Can you work these out from the model? Positions are in its coordinate system, mm. A direction names the side the tool comes from. Give positions to 0.01 mm unless a question says otherwise; leave off trailing zeros. Loops run counter-clockwise (first coordinate to the right, second up) from the corner with the lowest first, then second, coordinate; pieces in that order, holes last. Notation, with made-up numbers: (-4, 17) -> (15, 17) arc R8 cw to (15, 28) -> close; hole circle Ø5 at (-31.5, -15). An arc over 180 degrees is marked (long way). Use CSV: the item, a comma, the result in double quotes.
from build123d import *

# Parameters (mm, degrees)
F0_W     = 190
F0_H     = 60
F1_DEPTH = 5
F2_W     = 25
F2_H     = 20
F2_H_2   = 10
F2_W_2   = 24.9426496029
F3_DEPTH = 2
F4_W     = 25
F4_H     = 20
F4_H_2   = 10
F5_DEPTH = 2


with BuildPart() as f1:
    # F0 (on Top) → F1 (new body)
    with BuildSketch(Plane.XY):
        Rectangle(F0_W, F0_H)
        with BuildLine():
            Line((27, -16.5), (-27, -16.5))
            ThreePointArc((-27, -16.5), (-27.8535533906, -16.8535533906), (-27.5, -16))
            Line((-27.5, -16), (-27.5, -10))
            Line((-27.5, -10), (-42.4774698913, -10))
            Line((-42.4774698913, -10), (-42.4774698913, 10))
            Line((-42.4774698913, 10), (-27.5, 10))
            Line((-27.5, 10), (-27.5, 16))
            ThreePointArc((-27.5, 16), (-27.8535533906, 16.8535533906), (-27, 16.5))
            Line((-27, 16.5), (27, 16.5))
            ThreePointArc((27, 16.5), (27.5, 17), (28, 16.5))
            ThreePointArc((28, 16.5), (27.8535533906, 16.1464466094), (27.5, 16))
            Line((27.5, 16), (27.5, -16))
            ThreePointArc((27.5, -16), (27.8535533906, -16.1464466094), (28, -16.5))
            ThreePointArc((28, -16.5), (27.5, -17), (27, -16.5))
        make_face(mode=Mode.SUBTRACT)
        with BuildLine():
            ThreePointArc((-27.5, -16), (-27.1464466094, -16.1464466094), (-27, -16.5))
            Line((-27, -16.5), (27, -16.5))
            ThreePointArc((27, -16.5), (27.1464466094, -16.1464466094), (27.5, -16))
            Line((27.5, -16), (27.5, 16))
            ThreePointArc((27.5, 16), (27.1464466094, 16.1464466094), (27, 16.5))
            Line((27, 16.5), (-27, 16.5))
            ThreePointArc((-27, 16.5), (-27.1464466094, 16.1464466094), (-27.5, 16))
            Line((-27.5, 16), (-27.5, 10))
            Line((-27.5, 10), (-27.4774698913, 10))
            Line((-27.4774698913, 10), (-27.4774698913, -10))
            Line((-27.4774698913, -10), (-27.5, -10))
            Line((-27.5, -10), (-27.5, -16))
        make_face()
    extrude(amount=F1_DEPTH)

    # F2 (on face) → F3 (join)
    with BuildSketch(Plane.XY.offset(5)):
        Polygon((-95, -30), (-95, -20), (-95.0573503971, -20), (-95.0573503971, -50), (-70.0573503971, -50), (-70.0573503971, -30), align=None)
        with BuildLine():
            Line((-76.0573503971, -45), (-89.0573503971, -45))
            ThreePointArc((-89.0573503971, -45), (-90.7644571783, -45.7071067812), (-90.0573503971, -44))
            Line((-90.0573503971, -44), (-90.0573503971, -36))
            ThreePointArc((-90.0573503971, -36), (-90.7644571783, -34.2928932188), (-89.0573503971, -35))
            Line((-89.0573503971, -35), (-76.0573503971, -35))
            ThreePointArc((-76.0573503971, -35), (-75.0573503971, -34), (-74.0573503971, -35))
            ThreePointArc((-74.0573503971, -35), (-74.3502436159, -35.7071067812), (-75.0573503971, -36))
            Line((-75.0573503971, -36), (-75.0573503971, -44))
            ThreePointArc((-75.0573503971, -44), (-74.3502436159, -44.2928932188), (-74.0573503971, -45))
            ThreePointArc((-74.0573503971, -45), (-75.0573503971, -46), (-76.0573503971, -45))
        make_face(mode=Mode.SUBTRACT)
        with Locations((-82.5, 40)):
            Rectangle(F2_W, F2_H)
        with BuildLine():
            ThreePointArc((-90, 44), (-90.7071067812, 45.7071067812), (-89, 45))
            Line((-89, 45), (-76, 45))
            ThreePointArc((-76, 45), (-75, 46), (-74, 45))
            ThreePointArc((-74, 45), (-74.2928932188, 44.2928932188), (-75, 44))
            Line((-75, 44), (-75, 36))
            ThreePointArc((-75, 36), (-74.2928932188, 35.7071067812), (-74, 35))
            ThreePointArc((-74, 35), (-75, 34), (-76, 35))
            Line((-76, 35), (-89, 35))
            ThreePointArc((-89, 35), (-90.7071067812, 34.2928932188), (-90, 36))
            Line((-90, 36), (-90, 44))
        make_face(mode=Mode.SUBTRACT)
        with Locations((82.5, 40)):
            Rectangle(F2_W, F2_H)
        with BuildLine():
            ThreePointArc((75, 44), (74.2928932188, 45.7071067812), (76, 45))
            Line((76, 45), (89, 45))
            ThreePointArc((89, 45), (90, 46), (91, 45))
            ThreePointArc((91, 45), (90.7071067812, 44.2928932188), (90, 44))
            Line((90, 44), (90, 36))
            ThreePointArc((90, 36), (90.7071067812, 35.7071067812), (91, 35))
            ThreePointArc((91, 35), (90, 34), (89, 35))
            Line((89, 35), (76, 35))
            ThreePointArc((76, 35), (74.2928932188, 34.2928932188), (75, 36))
            Line((75, 36), (75, 44))
        make_face(mode=Mode.SUBTRACT)
        with Locations((82.5, -40)):
            Rectangle(F2_W, F2_H)
        with BuildLine():
            Line((89, -45), (76, -45))
            ThreePointArc((76, -45), (74.2928932188, -45.7071067812), (75, -44))
            Line((75, -44), (75, -36))
            ThreePointArc((75, -36), (74.2928932188, -34.2928932188), (76, -35))
            Line((76, -35), (89, -35))
            ThreePointArc((89, -35), (90, -34), (91, -35))
            ThreePointArc((91, -35), (90.7071067812, -35.7071067812), (90, -36))
            Line((90, -36), (90, -44))
            ThreePointArc((90, -44), (90.7071067812, -44.2928932188), (91, -45))
            ThreePointArc((91, -45), (90, -46), (89, -45))
        make_face(mode=Mode.SUBTRACT)
        with Locations((-82.5, 25)):
            Rectangle(F2_W, F2_H_2)
        with Locations((82.5, 25)):
            Rectangle(F2_W, F2_H_2)
        with Locations((82.5, -25)):
            Rectangle(F2_W, F2_H_2)
        with Locations((-82.5286751986, -25)):
            Rectangle(F2_W_2, F2_H_2)
        with BuildLine():
            Line((-76, 45), (-89, 45))
            ThreePointArc((-89, 45), (-89.2928932188, 44.2928932188), (-90, 44))
            Line((-90, 44), (-90, 36))
            ThreePointArc((-90, 36), (-89.2928932188, 35.7071067812), (-89, 35))
            Line((-89, 35), (-76, 35))
            ThreePointArc((-76, 35), (-75.7071067812, 35.7071067812), (-75, 36))
            Line((-75, 36), (-75, 44))
            ThreePointArc((-75, 44), (-75.7071067812, 44.2928932188), (-76, 45))
        make_face()
        with BuildLine():
            Line((89, 45), (76, 45))
            ThreePointArc((76, 45), (75.7071067812, 44.2928932188), (75, 44))
            Line((75, 44), (75, 36))
            ThreePointArc((75, 36), (75.7071067812, 35.7071067812), (76, 35))
            Line((76, 35), (89, 35))
            ThreePointArc((89, 35), (89.2928932188, 35.7071067812), (90, 36))
            Line((90, 36), (90, 44))
            ThreePointArc((90, 44), (89.2928932188, 44.2928932188), (89, 45))
        make_face()
        with BuildLine():
            ThreePointArc((75, -44), (75.7071067812, -44.2928932188), (76, -45))
            Line((76, -45), (89, -45))
            ThreePointArc((89, -45), (89.2928932188, -44.2928932188), (90, -44))
            Line((90, -44), (90, -36))
            ThreePointArc((90, -36), (89.2928932188, -35.7071067812), (89, -35))
            Line((89, -35), (76, -35))
            ThreePointArc((76, -35), (75.7071067812, -35.7071067812), (75, -36))
            Line((75, -36), (75, -44))
        make_face()
        with BuildLine():
            ThreePointArc((-90.0573503971, -44), (-89.3502436159, -44.2928932188), (-89.0573503971, -45))
            Line((-89.0573503971, -45), (-76.0573503971, -45))
            ThreePointArc((-76.0573503971, -45), (-75.7644571783, -44.2928932188), (-75.0573503971, -44))
            Line((-75.0573503971, -44), (-75.0573503971, -36))
            ThreePointArc((-75.0573503971, -36), (-75.7644571783, -35.7071067812), (-76.0573503971, -35))
            Line((-76.0573503971, -35), (-89.0573503971, -35))
            ThreePointArc((-89.0573503971, -35), (-89.3502436159, -35.7071067812), (-90.0573503971, -36))
            Line((-90.0573503971, -36), (-90.0573503971, -44))
        make_face()
    extrude(amount=F3_DEPTH)

    # F4 (on face) → F5 (join)
    with BuildSketch(Plane(origin=(0, 0, 0), x_dir=(1, 0, 0), z_dir=(0, 0, -1))):
        with Locations((-82.5, 40)):
            Rectangle(F4_W, F4_H)
        with BuildLine():
            ThreePointArc((-90, 44), (-90.7071067812, 45.7071067812), (-89, 45))
            Line((-89, 45), (-76, 45))
            ThreePointArc((-76, 45), (-75, 46), (-74, 45))
            ThreePointArc((-74, 45), (-74.2928932188, 44.2928932188), (-75, 44))
            Line((-75, 44), (-75, 36))
            ThreePointArc((-75, 36), (-74.2928932188, 35.7071067812), (-74, 35))
            ThreePointArc((-74, 35), (-75, 34), (-76, 35))
            Line((-76, 35), (-89, 35))
            ThreePointArc((-89, 35), (-90.7071067812, 34.2928932188), (-90, 36))
            Line((-90, 36), (-90, 44))
        make_face(mode=Mode.SUBTRACT)
        with Locations((82.5, 40)):
            Rectangle(F4_W, F4_H)
        with BuildLine():
            ThreePointArc((75, 44), (74.2928932188, 45.7071067812), (76, 45))
            Line((76, 45), (89, 45))
            ThreePointArc((89, 45), (90, 46), (91, 45))
            ThreePointArc((91, 45), (90.7071067812, 44.2928932188), (90, 44))
            Line((90, 44), (90, 36))
            ThreePointArc((90, 36), (90.7071067812, 35.7071067812), (91, 35))
            ThreePointArc((91, 35), (90, 34), (89, 35))
            Line((89, 35), (76, 35))
            ThreePointArc((76, 35), (74.2928932188, 34.2928932188), (75, 36))
            Line((75, 36), (75, 44))
        make_face(mode=Mode.SUBTRACT)
        with Locations((82.5, -40)):
            Rectangle(F4_W, F4_H)
        with BuildLine():
            Line((89, -45), (76, -45))
            ThreePointArc((76, -45), (74.2928932188, -45.7071067812), (75, -44))
            Line((75, -44), (75, -36.0721963992))
            ThreePointArc((75, -36.0721963992), (74.2928932188, -34.365089618), (76, -35.0721963992))
            Line((76, -35.0721963992), (89, -35.0721963992))
            ThreePointArc((89, -35.0721963992), (90, -34.0721963992), (91, -35.0721963992))
            ThreePointArc((91, -35.0721963992), (90.7071067812, -35.7793031804), (90, -36.0721963992))
            Line((90, -36.0721963992), (90, -44))
            ThreePointArc((90, -44), (90.7071067812, -44.2928932188), (91, -45))
            ThreePointArc((91, -45), (90, -46), (89, -45))
        make_face(mode=Mode.SUBTRACT)
        with Locations((-82.5, -40)):
            Rectangle(F4_W, F4_H)
        with BuildLine():
            Line((-76, -45), (-89, -45))
            ThreePointArc((-89, -45), (-90.7071067812, -45.7071067812), (-90, -44))
            Line((-90, -44), (-90, -36))
            ThreePointArc((-90, -36), (-90.7071067812, -34.2928932188), (-89, -35))
            Line((-89, -35), (-76, -35))
            ThreePointArc((-76, -35), (-75, -34), (-74, -35))
            ThreePointArc((-74, -35), (-74.2928932188, -35.7071067812), (-75, -36))
            Line((-75, -36), (-75, -44))
            ThreePointArc((-75, -44), (-74.2928932188, -44.2928932188), (-74, -45))
            ThreePointArc((-74, -45), (-75, -46), (-76, -45))
        make_face(mode=Mode.SUBTRACT)
        with Locations((-82.5, 25)):
            Rectangle(F4_W, F4_H_2)
        with Locations((82.5, 25)):
            Rectangle(F4_W, F4_H_2)
        with Locations((82.5, -25)):
            Rectangle(F4_W, F4_H_2)
        with Locations((-82.5, -25)):
            Rectangle(F4_W, F4_H_2)
        with BuildLine():
            Line((-76, 45), (-89, 45))
            ThreePointArc((-89, 45), (-89.2928932188, 44.2928932188), (-90, 44))
            Line((-90, 44), (-90, 36))
            ThreePointArc((-90, 36), (-89.2928932188, 35.7071067812), (-89, 35))
            Line((-89, 35), (-76, 35))
            ThreePointArc((-76, 35), (-75.7071067812, 35.7071067812), (-75, 36))
            Line((-75, 36), (-75, 44))
            ThreePointArc((-75, 44), (-75.7071067812, 44.2928932188), (-76, 45))
        make_face()
        with BuildLine():
            Line((89, 45), (76, 45))
            ThreePointArc((76, 45), (75.7071067812, 44.2928932188), (75, 44))
            Line((75, 44), (75, 36))
            ThreePointArc((75, 36), (75.7071067812, 35.7071067812), (76, 35))
            Line((76, 35), (89, 35))
            ThreePointArc((89, 35), (89.2928932188, 35.7071067812), (90, 36))
            Line((90, 36), (90, 44))
            ThreePointArc((90, 44), (89.2928932188, 44.2928932188), (89, 45))
        make_face()
        with BuildLine():
            ThreePointArc((-90, -44), (-89.2928932188, -44.2928932188), (-89, -45))
            Line((-89, -45), (-76, -45))
            ThreePointArc((-76, -45), (-75.7071067812, -44.2928932188), (-75, -44))
            Line((-75, -44), (-75, -36))
            ThreePointArc((-75, -36), (-75.7071067812, -35.7071067812), (-76, -35))
            Line((-76, -35), (-89, -35))
            ThreePointArc((-89, -35), (-89.2928932188, -35.7071067812), (-90, -36))
            Line((-90, -36), (-90, -44))
        make_face()
        with BuildLine():
            ThreePointArc((75, -44), (75.7071067812, -44.2928932188), (76, -45))
            Line((76, -45), (89, -45))
            ThreePointArc((89, -45), (89.2928932188, -44.2928932188), (90, -44))
            Line((90, -44), (90, -36.0721963992))
            ThreePointArc((90, -36.0721963992), (89.2928932188, -35.7793031804), (89, -35.0721963992))
            Line((89, -35.0721963992), (76, -35.0721963992))
            ThreePointArc((76, -35.0721963992), (75.7071067812, -35.7793031804), (75, -36.0721963992))
            Line((75, -36.0721963992), (75, -44))
        make_face()
    extrude(amount=F5_DEPTH)


solid = f1.part
(1) We'd pull the mould along Z, two halves only. Please class faces 4 (the face through (82, -40, 0)), 5 (the face through (-1, -30, 2)), 6 (the face through (82, 35, 7)), 7 (the face through (-95, -1, 3)): released by +Z, released by -Z, zero draft, split by the parting line, or undercut.
Answer sheet:
face 4,"undercut"
face 5,"undercut"
face 6,"released by +Z"
face 7,"zero draft"
(2) If we section it at B-B, the plane y = -28: Write out the boundary of the cut face in (x, z).
Answer sheet:
outline,"(-95.06, 5) -> (-95, 5) -> (-95, -2) -> (-70, -2) -> (-70, 0) -> (70, 0) -> (70, -2) -> (95, -2) -> (95, 7) -> (70, 7) -> (70, 5) -> (-70.06, 5) -> (-70.06, 7) -> (-95.06, 7) -> close"
(3) Will these pins go through, and if not, where does the flat tip stop? pin 1 Ø3 at (x, y) = (-90, 45) entering from +Z; pin 2 Ø3 at (x, y) = (-62, -1.5) entering from -Z; pin 3 Ø1.8 at (x, y) = (75, -45) entering from +Z; pin 4 Ø4 at (y, z) = (-2.5, 2) entering from -X.
Answer sheet:
pin 1,"stops at z = 7"
pin 2,"stops at z = 0"
pin 3,"passes through"
pin 4,"stops at x = -95"
(4) Which directions (+Z, -Z, +X, -X, +Y, -Y) give clear straight access to the entire face, cutting with the end or side of a thin tool? Please do faces 1 (the face through (-83, 40, 0)), 2 (the face through (82, -40, 5)), 3 (the face through (-35, 10, 2)).
Answer sheet:
face 1,"+X, -X, +Y"
face 2,"+X, -X, -Y"
face 3,"+Z, -Z"
(5) If we section it at C-C, the plane x = 37: Write out the boundary of the cut face in (y, z).
Answer sheet:
outline,"(-30, 0) -> (30, 0) -> (30, 5) -> (-30, 5) -> close"
(6) If I drill on L1, parallel to Y at x = -90, z = -1.15; L2, parallel to Y at x = 75, z = -1.5; L3, parallel to Z at x = -85, y = -40, over which ranges is the centre line in solid material (lowest first)? Write a range as from..to.
Answer sheet:
L1,"y = -50..-46, -44..-36, -34..-20, 20..34, 36..44, 46..50"
L2,"y = -50..-46, -44..-36, -34..-20, 20..34.07, 36.07..44, 46..50"
L3,"z = -2..0, 5..7"
(7) If we section it at A-A, the plane z = 2.75: Write out the boundary of the cut face in (x, y).
Answer sheet:
outline,"(-95, -30) -> (95, -30) -> (95, 30) -> (-95, 30) -> close; hole (-42.48, -10) -> (-27.48, -10) -> (-27.48, 10) -> (-42.48, 10) -> close; hole circle Ø1 at (-27.5, -16.5); hole circle Ø1 at (-27.5, 16.5); hole circle Ø1 at (27.5, -16.5); hole circle Ø1 at (27.5, 16.5)"
